Source: CAD feature listing. Evaluate the final solid. Frame: model axes, mm. Face numbers are marked on the shaded views. A direction names the side the tool comes from. Give positions to 0.01 mm unless a question says otherwise; leave off trailing zeros. Order: outer loops, then holes, each group sorted by start corner. A loop starts at its lowest first (then second) coordinate and runs counter-clockwise, first axis right, second up. Notation, with made-up numbers: M 49,20.25 L 99,20.25 A13 ccw 99,26.25 Z; hole C 43,-4 d7. An arc over 180 degrees is marked long. Use CSV: the item, a comma, the result in double quotes. Start each with the question number.
1. Section query D-D, the plane x = -2. Return the cut outline in (y, z), plus the area to 3 significant figures.
2. Section query B-B, the plane x = 0.7. Return the cut outline in (y, z).
3. Section query A-A, the plane y = 0. Return the cut outline in (x, z).
4. Pin query (flat end, axial travel): P1, Ø1, axis at x = 1, z = -23.5, coming from the +Y side; P2, Ø1.2, axis at x = 0.5, y = 0.5, coming from the +Z side; P3, Ø1.5, axis at x = -1.5, z = -12, coming from the +Y side. Return the tip coordinate at first contact, or that it passes through.
5. Section query C-C, the plane z = -15. Return the cut outline in (x, y), plus the area to 3 significant figures.
6. Reachability of the marked faces 1 and 2 from +Z, -Z, +X, -X, +Y, -Y: full face, straight path, thin tool, end or side. Return the list, or none.
7. Line query: line 1 along Y through (x, z) = (0.1, -9.5); line 2 along Z through (x, y) = (0.3, 0.65); line 3 along Z through (x, y) = (-1.95, -1.5). Output: solid intervals per line, ascending. Write a range as [from, to].
from build123d import *

# Parameters (mm, degrees)
SKETCH_1_R          = 2.75
EXTRUDE_1_DEPTH     = 3
CUT_EXTRUDE_1_DEPTH = 1.5
SKETCH_3_R          = 1.5
EXTRUDE_2_DEPTH     = 30


with BuildPart() as part:
    # 草图1 → 凸台-拉伸1 (new body)
    with BuildSketch(Plane.XY):
        Circle(SKETCH_1_R)
    extrude(amount=EXTRUDE_1_DEPTH)

    # 草图2 → 切除-拉伸1 (cut)
    with BuildSketch(Plane.XY.offset(3)):
        Polygon((0, -1.443375673), (1.25, -0.721687836), (1.25, 0.721687836), (0, 1.443375673), (-1.25, 0.721687836), (-1.25, -0.721687836), align=None)
    extrude(amount=-CUT_EXTRUDE_1_DEPTH, mode=Mode.SUBTRACT)

    # 草图3 → 凸台-拉伸2 (add)
    with BuildSketch(Plane(origin=(0, 0, 0), x_dir=(-1, 0, 0), z_dir=(0, 0, -1))):
        Circle(SKETCH_3_R)
    extrude(amount=EXTRUDE_2_DEPTH)


solid = part.part
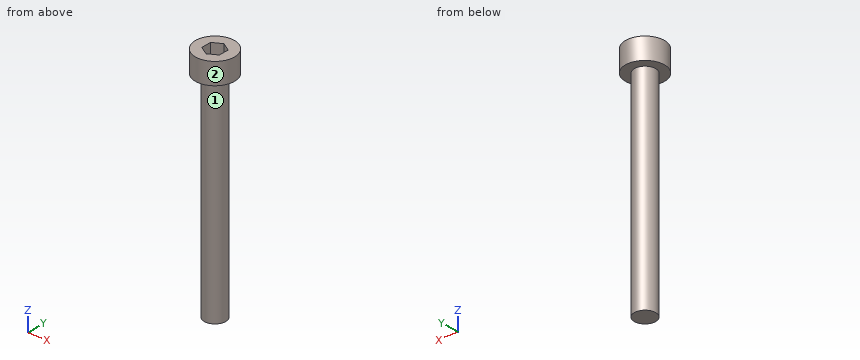
Result set:
1,outline,"M -1.89,0 L 1.89,0 L 1.89,3 L -1.89,3 Z"
1,area,"11.3 mm2"
2,outline,"M -2.66,0 L -1.33,0 L -1.33,-30 L 1.33,-30 L 1.33,0 L 2.66,0 L 2.66,3 L 1.04,3 L 1.04,1.5 L -1.04,1.5 L -1.04,3 L -2.66,3 Z"
3,outline,"M -2.75,0 L -1.5,0 L -1.5,-30 L 1.5,-30 L 1.5,0 L 2.75,0 L 2.75,3 L 1.25,3 L 1.25,1.5 L -1.25,1.5 L -1.25,3 L -2.75,3 Z"
4,P1,"y = 1.41"
4,P2,"z = 3"
4,P3,"y = 1.3"
5,outline,"C 0,0 d3"
5,area,"7.07 mm2"
6,face 1,"-Z"
6,face 2,"+Z, -Z"
7,line 1,"[-1.5, 1.5]"
7,line 2,"[-30, 1.5]"
7,line 3,"[0, 3]"
